Geometry check sheet. Reference: the model listing, model coordinates, mm. Round coordinates to 2 decimals unless told otherwise and drop trailing zeros. Write each loop counter-clockwise with the first axis right and the second up, starting at its lowest first coordinate (ties: lowest second). Pieces come first, ordered by that corner, then holes. Notation, with made-up numbers: M -9.5,6 L 26.5,6 A9 ccw 26.5,21 Z; hole C 36.5,62 d2. An arc over 180 degrees is marked long. Put each result on its own line as item: value. Start each with the question number.
(1) Section check C-C on x = -25. Record the cut outline in (y, z).
(2) Gauge pin test, flat ends, axial feed: pin 1 (0.6 mm diameter, centred on y = 1.5, z = -5, fed in from -X); pin 2 (3.5 mm diameter, centred on x = -35.36, z = 35.36, fed in from +Y); pin 3 (2 mm diameter, centred on x = 6.75, z = -40, fed in from -Y). Record the tip position at first contact, or that the pin passes through.
(3) Mould release check, pull along Z, two halves, no side actions. Record for faces 1 (the cylindrical face through (-0.07, 1.26, 51.5)), 2 (the flat face through (30, 6, 48)), 3 (the cylindrical face through (-26.76, 2.96, 51.46)): pulls with the +Z half, pulls with the -Z half, needs draft (parallel to the pull), parting line crosses it, or undercut.
(4) Section check B-B on y = 3.05. Record the cut outline in (x, z).
(5) Section check A-A on x = 0. Record the cut outline in (y, z).
(6) Material ranges on probe 1 along X at (y, z) = (1.75, 40); probe 2 along X at (y, z) = (1.4, 0); probe 3 along X at (y, z) = (1.05, 13.5), recorded low to high.
(7) Section check D-D on z = -32. Record the cut outline in (x, y).
Autodesk Inventor part; units mm, degrees
ref_plane "РабПлоскость6" through (-79.4555, 0, 0) normal (0, 0, -1) x (1, 0, 0)
ref_plane "РабПлоскость8" through (0, 7, 0) normal (0, -1, 0) x (1, 0, 0)
ref_plane "YZ Plane" through (0, 0, 0) normal (1, 0, 0) x (0, 1, 0)
sketch "Эскиз1" plane through (0, 0, 0) normal (0, 1, 0) x (-1, 0, 0)
  circle A0 centre (0, 0) radius 58
  line L0 (79.4555, 0) -> (-79.4555, 0)
  line L1 (0, -103.8803) -> (0, 88.3129)
  circle A1 centre (0, 0) radius 56
  line L2 (0, -103.8803) -> (0, 88.3129)
  line L3 (-79.4555, 0) -> (79.4555, 0)
  line L4 (11.5, -13.3) -> (23, -13.3)
  line L5 (23, -13.3) -> (23, 13.3)
  line L6 (23, 13.3) -> (11.5, 13.3)
  line L7 (11.5, 13.3) -> (11.5, -13.3)
  line L8 (35, -20) -> (45, -20)
  line L9 (45, -20) -> (45, 20)
  line L10 (45, 20) -> (35, 20)
  line L11 (35, 20) -> (35, -20)
  line L12 (17.25, -13.3) -> (17.25, 13.3)
  circle A2 centre (17.25, -9) radius 1
  circle A3 centre (17.25, 9) radius 1
  line L13 (3, 6) -> (33, 6)
  line L14 (33, 6) -> (33, -6)
  line L15 (33, -6) -> (3, -6)
  line L16 (3, -6) -> (3, 6)
  line L17 (-33, 6) -> (-33, -6)
  line L18 (-3, 6) -> (-33, 6)
  line L19 (-3, -6) -> (-3, 6)
  circle A4 centre (-17.25, 9) radius 1
  line L20 (-23, -13.3) -> (-23, 13.3)
  line L21 (-23, 13.3) -> (-11.5, 13.3)
  line L22 (-11.5, 13.3) -> (-11.5, -13.3)
  line L23 (-17.25, -13.3) -> (-17.25, 13.3)
  line L24 (-35, 20) -> (-35, -20)
  line L25 (-45, -20) -> (-45, 20)
  line L26 (-45, 20) -> (-35, 20)
  circle A5 centre (-17.25, -9) radius 1
  line L27 (-11.5, -13.3) -> (-23, -13.3)
  line L28 (-33, -6) -> (-3, -6)
  line L29 (-35, -20) -> (-45, -20)
  circle A6 centre (0, 0) radius 50
  circle A7 centre (0, -50) radius 1.5
  circle A8 centre (50, 0) radius 1.5
  circle A9 centre (0, 50) radius 1.5
  circle A10 centre (-50, 0) radius 1.5
  circle A11 centre (35.3553, -35.3553) radius 1.5
  circle A12 centre (50, 0) radius 1.5
  circle A13 centre (35.3553, 35.3553) radius 1.5
  circle A14 centre (0, 50) radius 1.5
  circle A15 centre (-35.3553, 35.3553) radius 1.5
  circle A16 centre (-50, 0) radius 1.5
  circle A17 centre (-35.3553, -35.3553) radius 1.5
  dimension "d0" = 116
  dimension "d135" = 11.5
  dimension "d136" = 26.6
  dimension "d137" = 10
  dimension "d138" = 40
  dimension "d139" = 45
  dimension "d140" = 12
  dimension "d141" = 2
  dimension "d142" = 18
  dimension "d143" = 2
  dimension "d144" = 30
  dimension "d145" = 12
  dimension "d146" = 2
  dimension "d147" = 100
  dimension "d148" = 3
  dimension "d149" = 3
  dimension "d150" = 3
  dimension "d151" = 3
  dimension "d152" = 360
  dimension "d168" = 112
extrude "Выдавливание1" add sketch "Эскиз1" along normal blind 6
sketch "Эскиз2" plane through (0, 0, 0) normal (0, -1, 0) x (1, 0, 0)
  circle A0 centre (0, 0) radius 57.5
  line L0 (0, -103.8803) -> (0, 88.3129)
  line L1 (-79.4555, 0) -> (79.4555, 0)
  circle A1 centre (0, 0) radius 50
  circle A2 centre (0, -50) radius 1.5
  circle A3 centre (50, 0) radius 1.5
  circle A4 centre (0, 50) radius 1.5
  circle A5 centre (-50, 0) radius 1.5
  circle A6 centre (35.3553, -35.3553) radius 1.5
  circle A7 centre (50, 0) radius 1.5
  circle A8 centre (35.3553, 35.3553) radius 1.5
  circle A9 centre (0, 50) radius 1.5
  circle A10 centre (-35.3553, 35.3553) radius 1.5
  circle A11 centre (-50, 0) radius 1.5
  circle A12 centre (-35.3553, -35.3553) radius 1.5
  circle A13 centre (0, 50) radius 2.8
  circle A14 centre (-11, 24) radius 1.5
  circle A15 centre (11, 24) radius 1.5
  circle A16 centre (11, -24) radius 1.5
  circle A17 centre (11, 24) radius 1.5
  circle A18 centre (-11, -24) radius 1.5
  circle A19 centre (-11, 24) radius 1.5
  circle A20 centre (50, 0) radius 1.5
  circle A21 centre (-50, 0) radius 1.5
  circle A22 centre (-17.25, -9) radius 1
  circle A23 centre (-35.3553, -35.3553) radius 1.5
  circle A24 centre (35.3553, 35.3553) radius 1.5
  circle A25 centre (35.3553, -35.3553) radius 1.5
  circle A26 centre (-35.3553, 35.3553) radius 1.5
  circle A27 centre (17.25, -9) radius 1
  circle A28 centre (17.25, 9) radius 1
  circle A29 centre (-17.25, 9) radius 1
  circle A30 centre (0, -50) radius 1.5
  circle A31 centre (0, 50) radius 1.5
  line L2 (0, 103.8803) -> (0, -88.3129)
  line L3 (-79.4555, 0) -> (79.4555, 0)
  circle A32 centre (6.75, 40) radius 1.15
  circle A33 centre (-6.75, 40) radius 1.15
  circle A34 centre (6.75, -40) radius 1.15
  circle A35 centre (-6.75, -40) radius 1.15
  circle A36 centre (0, 0) radius 56
  dimension "d22" = 3
  dimension "d23" = 3
  dimension "d26" = 3
  dimension "d30" = 360
  dimension "d84" = 115
  dimension "d118" = 5.6
  dimension "d155" = 2.3
  dimension "d156" = 13.5
  dimension "d157" = 10
  dimension "d158" = 2.3
  dimension "d159" = 13.5
  dimension "d160" = 10
sketch "Эскиз6" plane through (0, 6, 0) normal (0, 1, 0) x (1, 0, 0)
  circle A0 centre (0, 0) radius 58
  circle A1 centre (0, 0) radius 56
  dimension "d85" = 116
ref_plane "РабПлоскость6" through (-79.4555, 0, 0) normal (0, 0, -1) x (1, 0, 0)
ref_plane "РабПлоскость8" through (0, 7, 0) normal (0, -1, 0) x (1, 0, 0)
sketch "Эскиз11" plane through (0, 7, 0) normal (0, -1, 0) x (1, 0, 0)
  circle A0 centre (0, 0) radius 56
  dimension "d173" = 112
hole "Отверстие1" at (35.3553, 0, 35.3553) direction (0, 1, 0) diameter 3 end through all countersink diameter 4 countersink angle 90
hole "Отверстие2" at (0, 0, 50) at (-35.3553, 0, 35.3553) at (-50, 0, 0) at (-35.3553, 0, -35.3553) at (0, 0, -50) at (35.3553, 0, -35.3553) at (50, 0, 0) direction (0, 1, 0) diameter 3 end through all countersink diameter 4 countersink angle 90
extrude "Выдавливание15" cut sketch "Эскиз1" along normal through all contours L9 L8 L11 L0 | L0 L11 L10 L9 | L25 L26 L24 L0 | L0 L24 L29 L25
hole "Отверстие3" at (6.75, 0, -40) at (-6.75, 0, -40) at (6.75, 0, 40) at (-6.75, 0, 40) at (-17.25, 0, -9) at (-17.25, 0, 9) at (17.25, 0, -9) at (17.25, 0, 9) direction (0, 1, 0) diameter 1.567 end through all countersink diameter 3.8 countersink angle 90
extrude "Выдавливание17" cut sketch "Эскиз11" along normal blind 5
sketch "Эскиз13" plane through (0, 6, 0) normal (0, 1, 0) x (1, 0, 0)
  point P0 (0, 0)
properties part number "caseBottom" material "Пластик АБС"
Answers follow:
1. outline: M 0,-52.34 L 6,-52.34 L 6,-50.11 L 2,-50.11 L 2,50.11 L 6,50.11 L 6,52.34 L 0,52.34 Z
2. pin 1: stops at x = -57.81
2. pin 2: stops at y = 2
2. pin 3: stops at y = 0.9
3. face 1: undercut
3. face 2: needs draft
3. face 3: parting line crosses it
4. outline: C 0,0 d116; hole C 0,0 d112
5. outline: M 0,-58 L 6,-58 L 6,-56 L 2,-56 L 2,-51.5 L 0.5,-51.5 L 0,-52 Z; M 0,-48 L 0.5,-48.5 L 2,-48.5 L 2,48.5 L 0.5,48.5 L 0,48 Z; M 0,52 L 0.5,51.5 L 2,51.5 L 2,56 L 6,56 L 6,58 L 0,58 Z
6. probe 1: x = -42 to -7.53, -5.97 to 5.97, 7.53 to 42
6. probe 2: x = -58 to -51.5, -48.5 to -45, -35 to 35, 45 to 48.5, 51.5 to 58
6. probe 3: x = -56.41 to -45, -35 to 35, 45 to 56.41
7. outline: M -48.37,0 L 48.37,0 L 48.37,6 L 45.96,6 L 45.96,2 L -45.96,2 L -45.96,6 L -48.37,6 Z
